from build123d import *

# Parameters (mm, degrees)
F1_DEPTH = 10.16
F2_R     = 5.07999


# Not quite as in the source:
# - a fillet or chamfer is up to 0.001 mm smaller than in the source, because OpenCascade refuses the exact size


with BuildPart() as f1:
    # F0 (on Front) → F1 (new body)
    with BuildSketch(Plane.XZ):
        Polygon((-12.9241171581, 0), (0, 0), (0, 25.4), align=None)
    extrude(amount=F1_DEPTH)

    # F2 (radius 5.08 in the source; OpenCascade refuses exactly that, so slightly less here)
    f2_edges = [f1.edges().sort_by_distance(p)[0] for p in [
        (-6.462059, 0, 12.7),
        (-6.462059, -10.16, 12.7),
        (0, 0, 12.7),
        (0, -10.16, 12.7),
    ]]
    fillet(f2_edges, radius=F2_R)


solid = f1.part
Work out the finished part from the listing and answer in its coordinate system (mm). Give positions to 0.01 mm unless a question says otherwise; leave off trailing zeros. Loops run counter-clockwise (first coordinate to the right, second up) from the corner with the lowest first, then second, coordinate; pieces in that order, holes last. Notation, with made-up numbers: (-25.5, 17) - (5.5, 17) arc R24 cw to (5.5, 27) - close; hole circle Ø3 at (80.5, 15.5). An arc over 180 degrees is marked (long way). Answer in a Markdown table with one row per item.
(1) Section B-B (y = -2.25) is taken. Give the vertices of the cut face in (x, z), and give its area (3 significant figures).
Results list:
| item | result |
|---|---|
| outline | (-11.96, 0) - (-0.86, 0) - (-0.86, 21.81) - close |
| area | 121 mm² |
(2) Section A-A (y = -0.75) is taken. Give the vertices of the cut face in (x, z), and give its area (3 significant figures).
Results list:
| item | result |
|---|---|
| outline | (-10.21, 0) - (-2.42, 0) - (-2.42, 15.29) - close |
| area | 59.5 mm² |
(3) Flat-ended cylindrical pins translate along their axes: pin 1 Ø1.5 at (y, z) = (-3.5, 19.5) entering from -X; pin 2 Ø1 at (x, y) = (-9.5, -2) entering from +Z; pin 3 Ø1 at (y, z) = (-7.5, 6) entering from +X. Find the tip coordinate at first contact, or state that the pin passes through.
Results list:
| item | result |
|---|---|
| pin 1 | stops at x = -3.17 |
| pin 2 | stops at z = 5.69 |
| pin 3 | stops at x = -0.38 |
(4) Consider L1, parallel to Z at x = -9.75, y = -1.5; L2, parallel to Z at x = -8.25, y = -2.75; L3, parallel to X at y = -5.75, z = 4.5. Determine where each line is inside the solid, lowest interval first. Write a range as [from, to].
Results list:
| item | result |
|---|---|
| L1 | z = [0, 2.98] |
| L2 | z = [0, 7.94] |
| L3 | x = [-10.58, -0.04] |
